Autodesk Inventor part; units mm, degrees
ref_plane "作業平面1" through (50, 0, 0) normal (1, 0, 0) x (0, 1, 0)
ref_plane "作業平面2" through (-50, 0, 0) normal (1, 0, 0) x (0, 1, 0)
ref_plane "作業平面3" through (0, 50, 0) normal (0, 1, 0) x (-1, 0, 0)
sketch "スケッチ1" plane through (0, 0, 0) normal (0, 0, 1) x (1, 0, 0)
  circle A0 centre (0, 0) radius 50
  dimension "d0" = 100
extrude "押し出し1" add sketch "スケッチ1" along normal blind 8
ref_plane "作業平面1" through (50, 0, 0) normal (1, 0, 0) x (0, 1, 0)
ref_plane "作業平面2" through (-50, 0, 0) normal (1, 0, 0) x (0, 1, 0)
ref_plane "作業平面3" through (0, 50, 0) normal (0, 1, 0) x (-1, 0, 0)
ref_plane "作業平面4" through (0, -50, 0) normal (0, 1, 0) x (-1, 0, 0)
sketch "スケッチ2" plane through (50, 0, 0) normal (1, 0, 0) x (0, 1, 0)
  line L0 (0, 0) -> (0, 4) construction
  circle A0 centre (0, 4) radius 1.5
  dimension "d7" = 4
  dimension "d8" = 3
extrude "押し出し2" cut sketch "スケッチ2" against normal blind 5
sketch "スケッチ3" plane through (-50, 0, 0) normal (1, 0, 0) x (0, 1, 0)
  line L0 (0, 0) -> (0, 4) construction
  circle A0 centre (0, 4) radius 1.5
  dimension "d11" = 4
  dimension "d12" = 3
extrude "押し出し3" cut sketch "スケッチ3" along normal blind 5
sketch "スケッチ4" plane through (0, 50, 0) normal (0, 1, 0) x (-1, 0, 0)
  line L0 (0, 0) -> (0, 4) construction
  circle A0 centre (0, 4) radius 1.5
  dimension "d15" = 4
  dimension "d16" = 3
extrude "押し出し4" cut sketch "スケッチ4" against normal blind 5
sketch "スケッチ5" plane through (0, -50, 0) normal (0, 1, 0) x (-1, 0, 0)
  line L0 (0, 0) -> (0, 4) construction
  circle A0 centre (0, 4) radius 1.5
  dimension "d19" = 4
  dimension "d20" = 3
extrude "押し出し5" cut sketch "スケッチ5" along normal blind 5
thread "ねじ1"
thread "ねじ2"
thread "ねじ3"
thread "ねじ4"
sketch "スケッチ8" plane through (0, 0, 8) normal (0, 0, 1) x (1, 0, 0)
  line L0 (0, 0) -> (18.5, 0) construction
  line L1 (0, 0) -> (-18.5, 0) construction
  circle A0 centre (18.5, 0) radius 2
  circle A1 centre (-18.5, 0) radius 2
  circle A2 centre (0, 0) radius 6.5
  dimension "d62" = 18.5
  dimension "d63" = 18.5
  dimension "d64" = 4
  dimension "d65" = 4
  dimension "d66" = 13
extrude "押し出し7" cut sketch "スケッチ8" against normal blind 8
thread "ねじ7"
thread "ねじ8"
sketch "スケッチ9" plane through (0, 0, 8) normal (0, 0, 1) x (1, 0, 0)
  line L0 (0, 0) -> (25, 0) construction
  line L1 (25, 0) -> (25, -1) construction
  line L2 (25, 0) -> (25, 7.5) construction
  circle A0 centre (36, 7.5) radius 1
  line L3 (36, 7.5) -> (14, 7.5) construction
  circle A1 centre (14, 7.5) radius 1
  line L4 (25, -1) -> (25, -10) construction
  line L5 (25, -10) -> (25, -23) construction
  line L6 (25, 0) -> (9, 0) construction
  line L7 (9, 0) -> (9, -31) construction
  line L8 (9, -31) -> (41, -31) construction
  line L9 (41, -31) -> (41, 0) construction
  line L10 (25, 0) -> (25, 12) construction
  line L11 (14.417, 12) -> (35.583, 12) construction
  arc A2 (14.757, 12.2915) -> (9, 0) centre (25, 0) ccw construction
  arc A3 (41, 0) -> (35.583, 12) centre (25, 0) ccw construction
  line L12 (25, -10) -> (11.5, -10) construction
  line L13 (25, -23) -> (38.5, -23) construction
  circle A4 centre (11.5, -10) radius 1
  circle A5 centre (38.5, -23) radius 1
  dimension "d92" = 25
  dimension "d103" = 7.5
  dimension "d105" = 2
  dimension "d108" = 2
  dimension "d109" = 17.5
  dimension "d112" = 13
  dimension "d129" = 16
  dimension "d130" = 31
  dimension "d131" = 32
  dimension "d134" = 22
  dimension "d135" = 13.5
  dimension "d136" = 13.5
  dimension "d137" = 2
  dimension "d138" = 2
extrude "押し出し10" cut sketch "スケッチ9" against normal blind 8
properties part number "outsideCover"
Work out the finished part from the listing and answer in its coordinate system (mm). A direction names the side the tool comes from. Round coordinates to 2 decimals unless told otherwise and drop trailing zeros. Order: outer loops, then holes, each group sorted by start corner. A loop starts at its lowest first (then second) coordinate and runs counter-clockwise, first axis right, second up. Notation, with made-up numbers: M 53,53 L 80,53 A6 ccw 80,58 Z; hole C 87.5,-6 d3. An arc over 180 degrees is marked long. Put each result on its own line as item: value. Start each with the question number.
Q1. Section A-A, the plane y = 0 is taken. Write down the section's boundary in (x, z).
Q2. Section B-B, the plane x = -18.5 is taken. Write down the section's boundary in (y, z), and give its area (3 significant figures).
Q3. For a pull along Z with two mould halves and no side action, classify faces 6 (the flat face through (-1, -10, 8)), 7 (the cylindrical face through (-20.1, -1.2, 4.1)), 8 (the flat face through (45, 0, 4)) as pulls with the +Z half, pulls with the -Z half, needs draft (parallel to the pull), parting line crosses it, or undercut.
Q4. Straight lines are drawn through the part: L1, parallel to Z at x = 0, y = -46.65; L2, parallel to X at y = 4.5, z = 3; L3, parallel to Y at x = -2, z = 2.5. For each, find the intervals that lie inside material, in ascending order. Write a range as [from, to].
Q5. Flat-ended cylindrical pins translate along their axes: pin 1 (3 mm diameter, centred on y = 25.5, z = 2, fed in from +X); pin 2 (2.5 mm diameter, centred on x = 0, z = 4, fed in from -Y); pin 3 (1.8 mm diameter, centred on y = 0, z = 4, fed in from +X). Find the tip coordinate at first contact, or state that the pin passes through.
Q6. A tool of negligible diameter and unlimited length cuts with its end or side. For faces 1 (the cylindrical face through (47.535, 0.806, 5.265)), 2 (the flat face through (0, 45, 4)), 3 (the cylindrical face through (0.195, -47.535, 2.513)), 4 (the flat face through (-1, -10, 0)), 5 (the cylindrical face through (-47.535, 0.806, 2.735)), from which of +Z, -Z, +X, -X, +Y, -Y can it reach the whole face along a straight path? Write none if from no direction.
Q7. Section C-C, the plane x = 26.5 is taken. Write down the section's boundary in (y, z).
Q8. Section D-D, the plane y = 35 is taken. Write down the section's boundary in (x, z), and give its area (3 significant figures).
Findings below:
1. outline: M -50,0 L -20.5,0 L -20.5,8 L -50,8 L -50,5.5 L -45,5.5 L -45,2.5 L -50,2.5 Z; M -16.5,0 L -6.5,0 L -6.5,8 L -16.5,8 Z; M 6.5,0 L 16.5,0 L 16.5,8 L 6.5,8 Z; M 20.5,0 L 50,0 L 50,2.5 L 45,2.5 L 45,5.5 L 50,5.5 L 50,8 L 20.5,8 Z
2. outline: M -46.45,0 L -2,0 L -2,8 L -46.45,8 Z; M 2,0 L 46.45,0 L 46.45,8 L 2,8 Z
2. area: 711 mm^2
3. face 6: pulls with the +Z half
3. face 7: needs draft
3. face 8: undercut
4. L1: z = [0, 2.5], [5.5, 8]
4. L2: x = [-49.8, -4.69], [4.69, 49.8]
4. L3: y = [-49.96, -6.18], [6.18, 49.96]
5. pin 1: stops at x = 43.86
5. pin 2: stops at y = -45
5. pin 3: stops at x = 45
6. face 1: +X
6. face 2: +Y
6. face 3: -Y
6. face 4: -Z, +X, -X, +Y, -Y
6. face 5: -X
7. outline: M -42.4,0 L 42.4,0 L 42.4,8 L -42.4,8 Z
8. outline: M -35.71,0 L 35.71,0 L 35.71,8 L -35.71,8 Z
8. area: 571 mm^2
